Work out the finished part from the listing and answer in its coordinate system (mm). A direction names the side the tool comes from. Coordinates: 2 decimals unless noted, no trailing zeros. Order: outer loops, then holes, each group sorted by start corner. A loop starts at its lowest first (then second) coordinate and runs counter-clockwise, first axis right, second up.
1. The part is cut by section C-C, the plane y = 15. Count the separate pieces of the cut face and the enclosed holes in it, then the cut area to 3 significant figures.
2. Find the intervals of material crossed by probe 1 along Y at (x, z) = (-23, 2.85); probe 2 along Y at (x, z) = (0, 7); probe 3 along Y at (x, z) = (-8.5, 2.25), in increasing order.
3. Flat-ended cylindrical pins translate along their axes: pin 1 Ø5.5 at (x, y) = (23, 15) entering from +Z; pin 2 Ø3 at (x, z) = (-5.5, 6) entering from +Y. Find the tip coordinate at first contact, or state that the pin passes through.
4. Determine the mould class of faces 4 (the flat face through (-13, 5, 0)), 5 (the cylindrical face through (-28.14, 21.6, 1.52)), 6 (the cylindrical face through (-24.29, 17.024, 1.972)) for opening direction Y: +Y half, -Y half, draft (parallel to the pull), parting line (faces both ways), or undercut.
5. A tool of negligible diameter and unlimited length cuts with its end or side. For faces 1 (the flat face through (-25, 0, 4)), 2 (the flat face through (24, 0, 4)), 3 (the cylindrical face through (15.24, -6.32, 5.97)), from which of +Z, -Z, +X, -X, +Y, -Y can it reach the whole face along a straight path? Write none if from no direction.
6. The part is cut by section B-B, the plane x = -23.5. Give the vertices of the cut face in (y, z), then the cut area to 3 significant figures.
```python
from build123d import *

# Parameters (mm, degrees)
SKETCH1_W            = 58
SKETCH1_H            = 45
SKETCH1_R            = 2
BOSS_EXTRUDE1_DEPTH  = 4
SKETCH4_R            = 19.5
SKETCH4_R_2          = 16.5
BOSS_EXTRUDE3_DEPTH  = 4
SKETCH5_R            = 13.5
CUT_EXTRUDE2_DEPTH   = 37.922215535
M4_CLEARANCE_HOLE1_D = 4.8
FILLET1_R            = 3
FILLET2_R            = 1


with BuildPart() as part:
    # Sketch1 → Boss-Extrude1 (new body)
    # profile 1 of 5: a face of its own
    with BuildSketch(Plane.XY):
        Rectangle(SKETCH1_W, SKETCH1_H)
        with Locations((23, 15)):
            Circle(SKETCH1_R, mode=Mode.SUBTRACT)
        with Locations((23, -15)):
            Circle(SKETCH1_R, mode=Mode.SUBTRACT)
        with Locations((-23, -15)):
            Circle(SKETCH1_R, mode=Mode.SUBTRACT)
        with Locations((-23, 15)):
            Circle(SKETCH1_R, mode=Mode.SUBTRACT)
    # profile 2 of 5: a face of its own
    with BuildSketch(Plane.XY):
        with Locations((-23, 15)):
            Circle(SKETCH1_R)
    # profile 3 of 5: a face of its own
    with BuildSketch(Plane.XY):
        with Locations((-23, -15)):
            Circle(SKETCH1_R)
    # profile 4 of 5: a face of its own
    with BuildSketch(Plane.XY):
        with Locations((23, -15)):
            Circle(SKETCH1_R)
    # profile 5 of 5: a face of its own
    with BuildSketch(Plane.XY):
        with Locations((23, 15)):
            Circle(SKETCH1_R)
    extrude(amount=BOSS_EXTRUDE1_DEPTH)

    # Sketch4 → Boss-Extrude3 (add)
    with BuildSketch(Plane.XY.offset(4)):
        Circle(SKETCH4_R)
        Circle(SKETCH4_R_2, mode=Mode.SUBTRACT)
    extrude(amount=BOSS_EXTRUDE3_DEPTH)

    # Sketch5 → Cut-Extrude2 (cut, through all)
    with BuildSketch(Plane.XY.offset(4)):
        Circle(SKETCH5_R)
    extrude(amount=-CUT_EXTRUDE2_DEPTH, mode=Mode.SUBTRACT)

    # M4 Clearance Hole1 (through all)
    with Locations(Plane.XY.offset(4)):
        with Locations((23, 15), (23, -15), (-23, -15), (-23, 15)):
            Hole(M4_CLEARANCE_HOLE1_D / 2)

    # Fillet1
    fillet1_edges = [part.edges().sort_by_distance(p)[0] for p in [
        (-19.5, 0, 4),
        (29, -22.5, 2),
        (-29, -22.5, 2),
        (-29, 22.5, 2),
        (29, 22.5, 2),
    ]]
    fillet(fillet1_edges, radius=FILLET1_R - 0.0001)  # a hair under: the kernel refuses the full size

    # Fillet2
    fillet2_edges = [part.edges().sort_by_distance(p)[0] for p in [
        (-19.5, 0, 8),
        (0, -22.5, 4),
        (0, -22.5, 4),
        (-29, 0, 4),
        (29, 0, 4),
        (0, 22.5, 4),
        (0, 22.5, 4),
        (28.121349633, 21.621349633, 4),
        (28.121349633, -21.621349633, 4),
        (-28.121349633, 21.621349633, 4),
        (-28.121349633, -21.621349633, 4),
    ]]
    fillet(fillet2_edges, radius=FILLET2_R)


solid = part.part
```
Geometry says:
1. separate pieces: 3
1. enclosed holes: 0
1. area: 243 mm2
2. probe 1: y = -22.5 to -17.4, -12.6 to 12.6, 17.4 to 22.5
2. probe 2: y = -19.5 to -16.5, 16.5 to 19.5
2. probe 3: y = -22.5 to -10.49, 10.49 to 22.5
3. pin 1: stops at z = 4
3. pin 2: stops at y = 20.14
4. face 4: draft
4. face 5: +Y half
4. face 6: undercut
5. face 1: +Z, -X
5. face 2: +Z, +X
5. face 3: +Z
6. outline: (-22.5, 0) - (-17.35, 0) - (-17.35, 4) - (-21.5, 4) arc R1 ccw to (-22.5, 3) - close; (-12.65, 0) - (12.65, 0) - (12.65, 4) - (-12.65, 4) - close; (17.35, 0) - (22.5, 0) - (22.5, 3) arc R1 ccw to (21.5, 4) - (17.35, 4) - close
6. area: 142 mm2
